from build123d import *

# Parameters (mm, degrees)
SKETCH1_R           = 2.73935274
BOSS_EXTRUDE1_DEPTH = 60
SKETCH17_R          = 2.1
SKETCH17_W          = 39.9
SKETCH17_H          = 19.7
CUT_EXTRUDE10_DEPTH = 158.954623162
CUT_EXTRUDE11_DEPTH = 159.304157008
SKETCH19_W          = 123.088854382
SKETCH19_H          = 22
CUT_EXTRUDE12_DEPTH = 159.304157008
CUT_EXTRUDE14_DEPTH = 151.975703271
FILLET3_R           = 10
FILLET4_R           = 10
SKETCH16_R          = 2.1
SKETCH16_W          = 39.9
SKETCH16_H          = 19.7
CUT_EXTRUDE15_DEPTH = 40


with BuildPart() as part:
    # Sketch1 → Boss-Extrude1 (new body)
    with BuildSketch(Plane.XY):
        with BuildLine():
            Line((-79.073756432, 38.59348199), (120.926243568, 38.59348199))
            ThreePointArc((120.926243568, 38.59348199), (140.926243568, 18.59348199), (120.926243568, -1.40651801))
            Line((120.926243568, -1.40651801), (-79.073756432, -1.40651801))
            ThreePointArc((-79.073756432, -1.40651801), (-99.073756432, 18.59348199), (-79.073756432, 38.59348199))
        make_face()
        with Locations((-79.073756432, 18.59348199)):
            Circle(SKETCH1_R, mode=Mode.SUBTRACT)
        with Locations((120.926243568, 18.59348199)):
            Circle(SKETCH1_R, mode=Mode.SUBTRACT)
    extrude(amount=BOSS_EXTRUDE1_DEPTH)

    # Sketch17 → Cut-Extrude10 (cut, through all)
    with BuildSketch(Plane.XY.offset(60)):
        with Locations((86.11509795, 23.51848199)):
            Circle(SKETCH17_R)
        with Locations((86.11509795, 13.66848199)):
            Circle(SKETCH17_R)
        with Locations((135.537389186, 23.51848199)):
            Circle(SKETCH17_R)
        with Locations((135.537389186, 13.66848199)):
            Circle(SKETCH17_R)
        with Locations((110.826243568, 18.59348199)):
            Rectangle(SKETCH17_W, SKETCH17_H)
    extrude(amount=-CUT_EXTRUDE10_DEPTH, mode=Mode.SUBTRACT)

    # Sketch18 → Cut-Extrude11 (cut, through all)
    with BuildSketch(Plane(origin=(0, -1.40651801, 0), x_dir=(-1, 0, 0), z_dir=(0, -1, 0))):
        Polygon((-140.926243568, -55), (-140.926243568, 0), (-40.926243568, 0), align=None)
        Polygon((99.073756432, -55), (99.073756432, 0), (-0.926243568, 0), align=None)
    extrude(amount=-CUT_EXTRUDE11_DEPTH, mode=Mode.SUBTRACT)

    # Sketch19 → Cut-Extrude12 (cut, through all)
    with BuildSketch(Plane(origin=(0, -1.40651801, 0), x_dir=(-1, 0, 0), z_dir=(0, -1, 0))):
        with Locations((-19.381816377, -11)):
            Rectangle(SKETCH19_W, SKETCH19_H)
    extrude(amount=-CUT_EXTRUDE12_DEPTH, mode=Mode.SUBTRACT)

    # Sketch22 → Cut-Extrude14 (cut, through all)
    with BuildSketch(Plane(origin=(0, 0, 22), x_dir=(-1, 0, 0), z_dir=(0, 0, -1))):
        with BuildLine():
            Line((-80.926243568, 38.59348199), (39.073756432, 38.59348199))
            ThreePointArc((39.073756432, 38.59348199), (-20.926243568, 26.070752838), (-80.926243568, 38.59348199))
        make_face()
        with BuildLine():
            Line((-80.926243568, -1.40651801), (39.073756432, -1.40651801))
            ThreePointArc((39.073756432, -1.40651801), (-20.926243568, 11.116211141), (-80.926243568, -1.40651801))
        make_face()
    extrude(amount=-CUT_EXTRUDE14_DEPTH, mode=Mode.SUBTRACT)

    # Fillet3
    fillet3_edges = [part.edges().sort_by_distance(p)[0] for p in [
        (80.926243568, 18.59348199, 22),
    ]]
    fillet(fillet3_edges, radius=FILLET3_R)

    # Fillet4
    fillet4_edges = [part.edges().sort_by_distance(p)[0] for p in [
        (-39.073756432, 18.59348199, 22),
    ]]
    fillet(fillet4_edges, radius=FILLET4_R)

    # Sketch16 → Cut-Extrude15 (cut)
    with BuildSketch(Plane.XY.offset(60)):
        with Locations((-93.68490205, 23.51848199)):
            Circle(SKETCH16_R)
        with Locations((-93.68490205, 13.66848199)):
            Circle(SKETCH16_R)
        with Locations((-44.262610814, 23.51848199)):
            Circle(SKETCH16_R)
        with Locations((-44.262610814, 13.66848199)):
            Circle(SKETCH16_R)
        with Locations((-68.973756432, 18.59348199)):
            Rectangle(SKETCH16_W, SKETCH16_H)
    extrude(amount=-CUT_EXTRUDE15_DEPTH, mode=Mode.SUBTRACT)


solid = part.part
Geometry: final body of the model. Coordinates: model frame, mm. A direction names the side the tool comes from. Give positions to 0.01 mm unless a question says otherwise; leave off trailing zeros. Order: outer loops, then holes, each group sorted by start corner. A loop starts at its lowest first (then second) coordinate and runs counter-clockwise, first axis right, second up. Notation, with made-up numbers: (-18, -13.5) - (12, -13.5) arc R10 cw to (12, -2.5) - close; hole circle Ø2 at (24, 0.25). An arc over 180 degrees is marked (long way). Use CSV: the item, a comma, the result in double quotes.
1. Access query for faces 4 (the face through (97, -1.407, 45)), 5 (the face through (-49.024, 18, 44)). Directions: +Z, -Z, +X, -X, +Y, -Y. A direction counts if a zero-diameter tool reaches every point of the face in a straight line with its end or side. Return the directions, or none.
Answers below:
face 4,"+Z, -Z, +X, -X, -Y"
face 5,"+Z, -Z"
2. Section query B-B (z = 36). Output: boundary loops of the cut face in (x, y).
Answers below:
outline,"(-64.53, -1.41) - (-39.07, -1.41) arc R150 cw to (80.93, -1.41) - (106.38, -1.41) - (106.38, 8.74) - (90.88, 8.74) - (90.88, 28.44) - (106.38, 28.44) - (106.38, 38.59) - (80.93, 38.59) arc R150 cw to (-39.07, 38.59) - (-64.53, 38.59) - (-64.53, 28.44) - (-49.02, 28.44) - (-49.02, 8.74) - (-64.53, 8.74) - close; hole circle Ø4.2 at (-44.26, 13.67); hole circle Ø4.2 at (-44.26, 23.52); hole circle Ø4.2 at (86.12, 13.67); hole circle Ø4.2 at (86.12, 23.52)"
3. Contact query for flat-ended pins moving along their axis: pin 1 (2.5 mm diameter, centred on x = -44.26, y = 13.67, fed in from +Z); pin 2 (1.5 mm diameter, centred on y = 7.5, z = 54, fed in from +X); pin 3 (6 mm diameter, centred on y = 27, z = 44, fed in from -X); pin 4 (3 mm diameter, centred on y = 23, z = 38.5, fed in from -X). Output: stop coordinate, or through.
Answers below:
pin 1,"through"
pin 2,"x = 138.04"
pin 3,"x = -83.86"
pin 4,"x = -49.02"
4. Section query D-D (y = 31.5). Output: boundary loops of the cut face in (x, z).
Answers below:
outline,"(-94.35, 52.4) - (-41.32, 23.24) arc R10 ccw to (-36.51, 22) - (-19.06, 22) - (-19.06, 60) - (-94.35, 60) - close; (60.92, 22) - (78.36, 22) arc R10 ccw to (83.18, 23.24) - (136.2, 52.4) - (136.2, 60) - (60.92, 60) - close"
5. Mould query, pull axis Y, two halves, no side actions, for faces 1 (the face through (80.811, 18.873, 22.306)), 2 (the face through (84.017, 23.611, 42.05)), 3 (the face through (-54, -1.407, 45)). Classes: +Y half, -Y half, draft (parallel to the pull), parting line (faces both ways), or undercut.
Answers below:
face 1,"draft"
face 2,"undercut"
face 3,"-Y half"
6. Section query A-A (y = 6.5). Output: boundary loops of the cut face in (x, z), plus the area to 3 significant figures.
Answers below:
outline,"(-95, 52.76) - (-41.32, 23.24) arc R10 ccw to (-36.51, 22) - (-16, 22) - (-16, 60) - (-95, 60) - close; (57.85, 22) - (78.36, 22) arc R10 ccw to (83.18, 23.24) - (136.86, 52.76) - (136.86, 60) - (57.85, 60) - close"
area,"4,280 mm2"
7. Material intervals for line 1 along X through (y, z) = (14, 41.5); line 2 along Y through (x, z) = (-67.5, 58); line 3 along X through (y, z) = (24.5, 49), sorted ascending. Write a range as from..to.
Answers below:
line 1,"-49.02..-46.34, -42.19..84.04, 88.19..90.88"
line 2,"-1.41..8.74, 28.44..38.59"
line 3,"-49.02..-46.12, -42.41..84.26, 87.97..90.88"
8. Section query C-C (x = 112). Output: boundary loops of the cut face in (y, z), plus the area to 3 significant figures.
Answers below:
outline,"(-1.41, 39.09) - (8.74, 39.09) - (8.74, 60) - (-1.41, 60) - close; (28.44, 39.09) - (38.59, 39.09) - (38.59, 60) - (28.44, 60) - close"
area,"424 mm2"
